```python
from build123d import *

# Parameters (mm, degrees)
EXTRUDE_1_DEPTH     = 20
RIB_1_REACH         = 57.283
SKETCH_2_WALL_W     = 155.769731092
SKETCH_2_WALL_H     = 4
HOLE_WIZARD_M4_1_D  = 3.3
SKETCH_6_R          = 2.5
CUT_EXTRUDE_1_DEPTH = 2.2
SKETCH_7_R          = 1
CUT_EXTRUDE_2_DEPTH = 10
FILLET_1_R          = 1
SKETCH_8_R          = 1.525
EXTRUDE_2_DEPTH     = 2.5
FILLET_2_R          = 3


with BuildPart() as part:
    # 草图1 → 凸台-拉伸1 (new, symmetric)
    with BuildSketch(Plane.XY):
        Polygon((0, 0), (20, 0), (20, -47.5), (17.5, -47.5), (17.5, -8), (0, -8), align=None)
    extrude(amount=EXTRUDE_1_DEPTH, both=True)

    # 草图2 wall → 筋1 (add, up to next)
    with BuildSketch(Plane(origin=(8.75, -27.75, 0), x_dir=(0.405064377285, -0.914288165872, 0), z_dir=(0.914288165872, 0.405064377285, 0)), mode=Mode.PRIVATE) as rib_1_sk1:
        Rectangle(SKETCH_2_WALL_W, SKETCH_2_WALL_H)
    rib_1_tool1 = extrude(rib_1_sk1.sketch, amount=RIB_1_REACH, mode=Mode.PRIVATE) - part.part
    add(rib_1_tool1.solids().sort_by_distance((8.75, -27.75, 0))[0])

    # M4 螺纹孔1 (through all)
    with Locations(Plane(origin=(0, -8, 0), x_dir=(-1, 0, 0), z_dir=(0, -1, 0))):
        with Locations((-4, 15), (-15, 15)):
            hole_wizard_m4_1 = Hole(HOLE_WIZARD_M4_1_D / 2)

    # 镜向1: M4 螺纹孔1 across plane
    add(hole_wizard_m4_1.mirror(Plane.XY), mode=Mode.SUBTRACT)

    # 草图6 → 切除-拉伸1 (cut)
    with BuildSketch(Plane(origin=(0, 0, 0), x_dir=(1, 0, 0), z_dir=(0, 1, 0))):
        with Locations(Location((15, 15, 0), (0, 0, 270))):
            Circle(SKETCH_6_R)
        with Locations(Location((4, 15, 0), (0, 0, 270))):
            Circle(SKETCH_6_R)
        with Locations(Location((4, -15, 0), (0, 0, 270))):
            Circle(SKETCH_6_R)
        with Locations(Location((15, -15, 0), (0, 0, 270))):
            Circle(SKETCH_6_R)
    extrude(amount=-CUT_EXTRUDE_1_DEPTH, mode=Mode.SUBTRACT)

    # 草图7 → 切除-拉伸2 (cut)
    with BuildSketch(Plane.ZY.offset(-17.5)):
        with Locations(Location((-5.5, -44.25, 0), (0, 0, 270))):
            Circle(SKETCH_7_R)
        with Locations(Location((-17.5, -44.25, 0), (0, 0, 270))):
            Circle(SKETCH_7_R)
        with Locations(Location((-5.5, -36.25, 0), (0, 0, 270))):
            Circle(SKETCH_7_R)
        with Locations(Location((-17.5, -36.25, 0), (0, 0, 270))):
            Circle(SKETCH_7_R)
        with Locations(Location((-5.5, -19.75, 0), (0, 0, 270))):
            Circle(SKETCH_7_R)
        with Locations(Location((-5.5, -11.75, 0), (0, 0, 270))):
            Circle(SKETCH_7_R)
        with Locations(Location((-17.5, -19.75, 0), (0, 0, 270))):
            Circle(SKETCH_7_R)
        with Locations(Location((-17.5, -11.75, 0), (0, 0, 270))):
            Circle(SKETCH_7_R)
        with Locations(Location((17.5, -11.75, 0), (0, 0, 270))):
            Circle(SKETCH_7_R)
        with Locations(Location((17.5, -19.75, 0), (0, 0, 270))):
            Circle(SKETCH_7_R)
        with Locations(Location((5.5, -11.75, 0), (0, 0, 270))):
            Circle(SKETCH_7_R)
        with Locations(Location((5.5, -19.75, 0), (0, 0, 270))):
            Circle(SKETCH_7_R)
        with Locations(Location((17.5, -36.25, 0), (0, 0, 270))):
            Circle(SKETCH_7_R)
        with Locations(Location((5.5, -36.25, 0), (0, 0, 270))):
            Circle(SKETCH_7_R)
        with Locations(Location((17.5, -44.25, 0), (0, 0, 270))):
            Circle(SKETCH_7_R)
        with Locations(Location((5.5, -44.25, 0), (0, 0, 270))):
            Circle(SKETCH_7_R)
    extrude(amount=-CUT_EXTRUDE_2_DEPTH, mode=Mode.SUBTRACT)

    # 圆角1
    fillet_1_edges = [part.edges().sort_by_distance(p)[0] for p in [
        (18.75, -47.5, 20),
        (0, -4, 20),
        (18.75, -47.5, -20),
        (0, -4, -20),
    ]]
    fillet(fillet_1_edges, radius=FILLET_1_R)

    # 草图8 → 凸台-拉伸2 (add)
    with BuildSketch(Plane.ZY.offset(-17.5)):
        with BuildLine():
            Line((19, -47.5), (25, -47.5))
            ThreePointArc((25, -47.5), (28, -44.5), (25, -41.5))
            Line((25, -41.5), (20, -41.5))
            Line((20, -41.5), (19, -47.5))
        make_face()
        with Locations((25, -44.5)):
            Circle(SKETCH_8_R, mode=Mode.SUBTRACT)
    extrude_2 = extrude(amount=-EXTRUDE_2_DEPTH)

    # 镜向2: 凸台-拉伸2 across plane
    add(extrude_2.mirror(Plane.XY))

    # 圆角2
    fillet_2_edges = [part.edges().sort_by_distance(p)[0] for p in [
        (18.75, -41.5, 20),
        (18.75, -41.5, -20),
    ]]
    fillet(fillet_2_edges, radius=FILLET_2_R)


solid = part.part
```
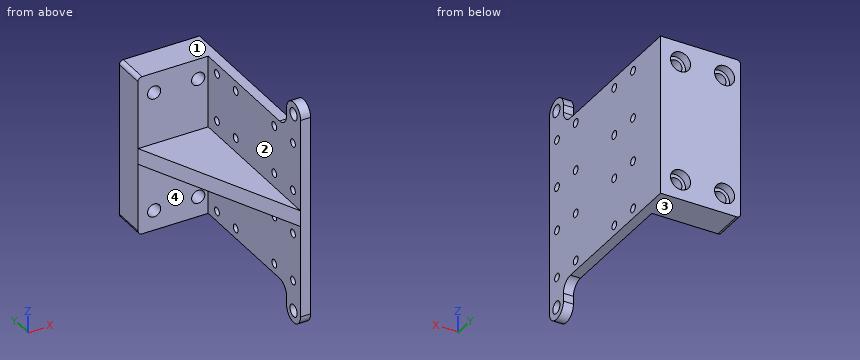
Model file for the job. Use its own axes, mm. Face numbers are marked on the shaded views. A direction names the side the tool comes from. Give positions to 0.01 mm unless a question says otherwise; leave off trailing zeros. Order: outer loops, then holes, each group sorted by start corner. A loop starts at its lowest first (then second) coordinate and runs counter-clockwise, first axis right, second up.
1) 3-axis set-ups, long thin cutter, end or side, ignore diameter. For the marked faces 1, 2, 3 and 4: which of +Z, -Z, +X, -X, +Y, -Y reach the whole face in a straight line?
2) Saw through at A-A, the plane z = 15. Write the cut outline in (x, y).
3) Saw through at D-D, the plane y = -36.25. Write the cut outline in (x, z).
4) Pin check, flat tips, straight feed: pin 1 (1.5 mm diameter, centred on y = -31, z = -1.5, fed in from -X); pin 2 (12 mm diameter, centred on x = 2, z = 15, fed in from -Y); pin 3 (1.5 mm diameter, centred on x = 3, z = -15, fed in from +Y). Stop position of each tip, or through.
5) Wall check: probe 1 along Z at (x, y) = (19.4, -11.75); probe 2 along X at (y, z) = (-7, 15); probe 3 along X at (y, z) = (-1.3, 15). Give the ranges that are in metal, low to high.
6) Saw through at B-B, the plane y = -44.5. Count the separate pieces of the cut face and the enclosed holes in it, then the cut area to 3 significant figures.
7) Saw through at C-C, the plane x = 15. Write the cut outline in (y, z).
Computed:
1. face 1: +Z, +X, -X, +Y
1. face 2: +Z, -X, -Y
1. face 3: -Z, +X, -X, +Y
1. face 4: -Z, -X, -Y
2. outline: (0, -8) - (2.35, -8) - (2.35, -2.2) - (1.5, -2.2) - (1.5, 0) - (0, 0) - close; (5.65, -8) - (13.35, -8) - (13.35, -2.2) - (12.5, -2.2) - (12.5, 0) - (6.5, 0) - (6.5, -2.2) - (5.65, -2.2) - close; (16.65, -8) - (17.5, -8) - (17.5, -47.5) - (20, -47.5) - (20, 0) - (17.5, 0) - (17.5, -2.2) - (16.65, -2.2) - close
3. outline: (12.52, -2) - (17.5, -2) - (17.5, -4.5) - (20, -4.5) - (20, 4.5) - (17.5, 4.5) - (17.5, 2) - (12.52, 2) - close; (17.5, -20) - (20, -20) - (20, -18.5) - (17.5, -18.5) - close; (17.5, -16.5) - (20, -16.5) - (20, -6.5) - (17.5, -6.5) - close; (17.5, 6.5) - (20, 6.5) - (20, 16.5) - (17.5, 16.5) - close; (17.5, 18.5) - (20, 18.5) - (20, 20) - (17.5, 20) - close
4. pin 1: stops at x = 9.86
4. pin 2: stops at y = -8
4. pin 3: stops at y = -2.2
5. probe 1: z = -20 to -18.5, -16.5 to -6.5, -4.5 to 4.5, 6.5 to 16.5, 18.5 to 20
5. probe 2: x = 0 to 2.35, 5.65 to 13.35, 16.65 to 20
5. probe 3: x = 0 to 1.5, 6.5 to 12.5, 17.5 to 20
6. separate pieces: 7
6. enclosed holes: 0
6. area: 111 mm2
7. outline: (-41.86, -2) - (-8, -2) - (-8, -13.35) - (-2.2, -13.35) - (-2.2, -12.5) - (0, -12.5) - (0, 12.5) - (-2.2, 12.5) - (-2.2, 13.35) - (-8, 13.35) - (-8, 2) - (-41.86, 2) - close; (-8, -20) - (0, -20) - (0, -17.5) - (-2.2, -17.5) - (-2.2, -16.65) - (-8, -16.65) - close; (-8, 16.65) - (-2.2, 16.65) - (-2.2, 17.5) - (0, 17.5) - (0, 20) - (-8, 20) - close
